The listing builds one solid part. Answer for the finished solid, in the listing's coordinates (mm). A direction names the side the tool comes from. Give positions to 0.01 mm unless a question says otherwise; leave off trailing zeros. Loops run counter-clockwise (first coordinate to the right, second up) from the corner with the lowest first, then second, coordinate; pieces in that order, holes last. Notation, with made-up numbers: M 22.5,51.25 L 55.5,51.25 A9 cw 55.5,64.25 Z; hole C -23,20 d3. An arc over 180 degrees is marked long. Use one line per item in the form item = value. Start each with the question number.
1. The part is cut by section D-D (x = 18.5). Write down the section's boundary in (y, z), and give its area (3 significant figures).
2. The part is cut by section A-A (x = 0). Write down the section's boundary in (y, z).
3. The mould has two halves that part along Y. Classify faces 5 (the face through (1, 254, -50)), 6 (the face through (-34.966, 85.445, 0.7)), 7 (the face through (-0.6, 310, 0.7)): released by +Y, released by -Y, zero draft, split by the parting line, or undercut.
4. Each of these flat-tipped pins is pushed along its axis until it touches: pin 1 Ø24 at (x, y) = (-19.5, 83.5) entering from +Z; pin 2 Ø5 at (x, z) = (28.5, 78) entering from +Y; pin 3 Ø5 at (x, y) = (18.5, 188.5) entering from -Z. Where does it stop, or does it pass through?
5. The part is cut by section C-C (y = 270). Write down the section's boundary in (x, z).
6. Straight lines are drawn through the part: line 1 (Y direction, x = 0, z = 2); line 2 (Y direction, x = -33, z = -39); line 3 (Y direction, x = 10, z = -12.5). For each, find the intervals that lie inside material, in ascending order. Write a range as from..to.
7. The part is cut by section B-B (z = -1.5). Write down the section's boundary in (x, y).
8. For faces 1 (the face through (1, 217.5, -54)), 2 (the face through (-30, 57, 1)), 3 (the face through (1, 93, 50)), 4 (the face through (40, 149, -3)), determine the directions among +Z, -Z, +X, -X, +Y, -Y from which every point of the face is accessible in a straight line to the end or side of a thin tool.
from build123d import *

# Parameters (mm, degrees)
SKETCH1_W           = 115
SKETCH1_H           = 210
BOSS_EXTRUDE1_DEPTH = 30
SKETCH2_W           = 60
SKETCH2_H           = 60
BOSS_EXTRUDE3_DEPTH = 50
SKETCH3_R           = 15
BOSS_EXTRUDE4_DEPTH = 50
SKETCH8_W           = 8
SKETCH8_H           = 45
BOSS_EXTRUDE7_DEPTH = 80
CUT_EXTRUDE1_DEPTH  = 180


with BuildPart() as part:
    # Sketch1 → Boss-Extrude1 (new body)
    with BuildSketch(Plane(origin=(0, 0, 0), x_dir=(1, 0, 0), z_dir=(0, 1, 0))):
        Rectangle(SKETCH1_W, SKETCH1_H)
    extrude(amount=BOSS_EXTRUDE1_DEPTH)

    # Sketch2 → Boss-Extrude3 (add, symmetric)
    with BuildSketch(Plane.XY):
        with Locations((0, 60)):
            Rectangle(SKETCH2_W, SKETCH2_H)
    extrude(amount=BOSS_EXTRUDE3_DEPTH, both=True)

    # Sketch3 → Boss-Extrude4 (add, symmetric)
    with BuildSketch(Plane.XY):
        with BuildLine():
            Line((-40, 87.180706736), (-40, 302.819293264))
            ThreePointArc((-40, 302.819293264), (0, 310), (40, 302.819293264))
            Line((40, 302.819293264), (40, 87.180706736))
            ThreePointArc((40, 87.180706736), (0, 80), (-40, 87.180706736))
        make_face()
        with Locations((0, 270)):
            Circle(SKETCH3_R, mode=Mode.SUBTRACT)
        with Locations((0, 120)):
            Circle(SKETCH3_R, mode=Mode.SUBTRACT)
    extrude(amount=BOSS_EXTRUDE4_DEPTH, both=True)

    # Sketch8 → Boss-Extrude7 (add)
    with BuildSketch(Plane(origin=(40, 0, 0), x_dir=(0, 0, -1), z_dir=(1, 0, 0))):
        with Locations((54, 195)):
            Rectangle(SKETCH8_W, SKETCH8_H)
    extrude(amount=-BOSS_EXTRUDE7_DEPTH)

    # Sketch7 → Cut-Extrude1 (cut)
    with BuildSketch(Plane.ZY.offset(40)):
        with BuildLine():
            Line((-10, 235), (50, 235))
            Line((50, 235), (50, 155))
            Line((50, 155), (-10, 155))
            ThreePointArc((-10, 155), (-50, 195), (-10, 235))
        make_face()
    extrude(amount=-CUT_EXTRUDE1_DEPTH, mode=Mode.SUBTRACT)


solid = part.part
Derived:
q1.outline = M 0,-105 L 30,-105 L 30,-50 L 172.5,-50 L 172.5,-58 L 217.5,-58 L 217.5,-50 L 308.5,-50 L 308.5,50 L 235,50 L 235,-10 A40 cw 155,-10 L 155,50 L 30,50 L 30,105 L 0,105 Z
q1.area = 27,200 mm2
q2.outline = M 0,-105 L 30,-105 L 30,-50 L 105,-50 L 105,50 L 30,50 L 30,105 L 0,105 Z; M 135,-50 L 172.5,-50 L 172.5,-58 L 217.5,-58 L 217.5,-50 L 255,-50 L 255,50 L 235,50 L 235,-10 A40 cw 155,-10 L 155,50 L 135,50 Z; M 285,-50 L 310,-50 L 310,50 L 285,50 Z
q3.face_5 = zero draft
q3.face_6 = undercut
q3.face_7 = released by +Y
q4.pin_1 = 50
q4.pin_2 = 30
q4.pin_3 = -58
q5.outline = M -40,-50 L -15,-50 L -15,50 L -40,50 Z; M 15,-50 L 40,-50 L 40,50 L 15,50 Z
q6.line_1 = 0..105, 135..155, 235..255, 285..310
q6.line_2 = 0..30, 84.84..167.45, 222.55..305.16
q6.line_3 = 0..108.82, 131.18..155.08, 234.92..258.82, 281.18..309.56
q7.outline = M -57.5,0 L 57.5,0 L 57.5,30 L 30,30 L 30,83.98 A115 ccw 40,87.18 L 40,155 L -40,155 L -40,87.18 A115 ccw -30,83.98 L -30,30 L -57.5,30 Z; M -40,235 L 40,235 L 40,302.82 A115 ccw -40,302.82 Z; hole C 0,120 d30; hole C 0,270 d30
q8.face_1 = -Z, +X, -X, +Y
q8.face_2 = +Z, -Z, -X
q8.face_3 = +Z, +X, -X, +Y
q8.face_4 = +Z, -Z, +X, +Y
